Build history of the part. All positions in model axes, mm. Face numbers are marked on the shaded views. A direction names the side the tool comes from. Coordinates: 2 decimals unless noted, no trailing zeros. Loops run counter-clockwise (first coordinate to the right, second up) from the corner with the lowest first, then second, coordinate; pieces in that order, holes last.
(1) Tool access for the marked faces 1, 2 and 3: list every direction of +Z, -Z, +X, -X, +Y, -Y with a clear straight run to the whole face (end or side of a thin tool).
(2) Wall check: L1, parallel to X at y = -52, z = -4; L2, parallel to Z at x = 43, y = -9.5; L3, parallel to Y at x = -4, z = -12.75. Give the ranges that are in metal, low to high.
(3) Flat gauge pins, fed straight in: P1, Ø6, axis at y = -30.5, z = -7.5, coming from the -X side; P2, Ø6.5, axis at y = 7.5, z = 3.5, coming from the -X side; P3, Ø4, axis at x = 3, z = -16.5, coming from the -Y side. Where does each tip first touch, or does it go through?
(4) Slice it at B-B (y = -33). Give the cut face in (x, z) (1 decimal), and give its area (3 significant figures).
(5) Slice it at A-A (x = 1). Give the cut face in (y, z).
(6) Slice it at C-C (z = 3.25). Give the cut face in (x, y) (3 decimals), and give its area (3 significant figures).
(7) Slice it at D-D (z = -16.25). Give the cut face in (x, y), and give its area (3 significant figures).
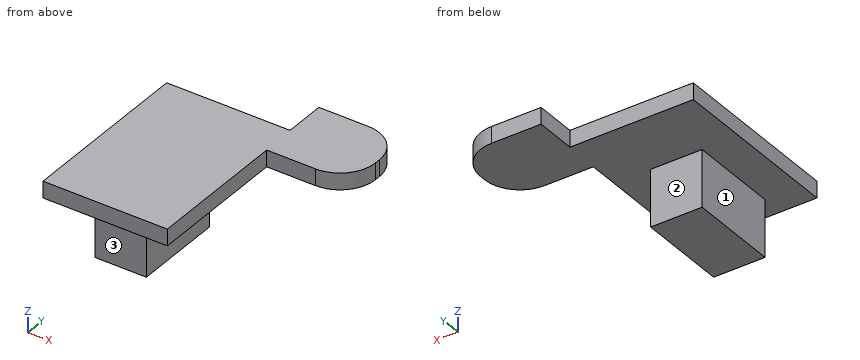
from build123d import *

# Parameters (mm, degrees)
F2_DEPTH = 5.9182
F0_W     = 44.45
F0_H     = 63.5
F3_DEPTH = 5.9182
F4_W     = 18.415
F4_H     = 32.385
F5_DEPTH = 20.32


with BuildPart() as f2:
    # F1 (on Top) → F2 (new body)
    with BuildSketch(Plane.XY):
        with BuildLine():
            Line((39.6100495338, 16.1036532372), (21.8759961426, 16.1036532372))
            Line((21.8759961426, 16.1036532372), (21.8759961426, -11.2066548318))
            Line((21.8759961426, -11.2066548318), (39.6100495338, -11.2066548318))
            ThreePointArc((39.6100495338, -11.2066548318), (48.5903056549, -7.4869109528), (52.3100495338, 1.4933451682))
            Line((52.3100495338, 1.4933451682), (52.3100495338, 3.4036532372))
            ThreePointArc((52.3100495338, 3.4036532372), (48.5903056549, 12.3839093583), (39.6100495338, 16.1036532372))
        make_face()
    extrude(amount=F2_DEPTH)

    # F0 (on Top) + F2_face (on face) → F3 (join)
    with BuildSketch(Plane.XY):
        with Locations((0, -30.48)):
            Rectangle(F0_W, F0_H)
    with BuildSketch(Plane(origin=(35.9682073334, 2.4484992027, 0), x_dir=(1, 0, 0), z_dir=(0, 0, -1))):
        with BuildLine():
            Line((-14.0922111908, -13.6551540345), (3.6418422005, -13.6551540345))
            ThreePointArc((3.6418422005, -13.6551540345), (12.6220983215, -9.9354101556), (16.3418422005, -0.9551540345))
            Line((16.3418422005, -0.9551540345), (16.3418422005, 0.9551540345))
            ThreePointArc((16.3418422005, 0.9551540345), (12.6220983215, 9.9354101556), (3.6418422005, 13.6551540345))
            Line((3.6418422005, 13.6551540345), (-14.0922111908, 13.6551540345))
            Line((-14.0922111908, 13.6551540345), (-14.0922111908, -13.6551540345))
        make_face()
    extrude(amount=F3_DEPTH, dir=(0, 0, 1))

    # F4 (on Top) → F5 (join)
    with BuildSketch(Plane.XY):
        with Locations((0, -38.1122922906)):
            Rectangle(F4_W, F4_H)
    extrude(amount=-F5_DEPTH)


solid = f2.part
Response values:
1. face 1: -Z, -X, +Y, -Y
1. face 2: -Z, +X, -X, +Y
1. face 3: -Z, +X, -X, -Y
2. L1: x = -9.21 to 9.21
2. L2: z = 0 to 5.92
2. L3: y = -54.3 to -21.92
3. P1: stops at x = -9.21
3. P2: stops at x = 21.88
3. P3: stops at y = -54.3
4. outline: (-22.2, 0) - (-9.2, 0) - (-9.2, -20.3) - (9.2, -20.3) - (9.2, 0) - (22.2, 0) - (22.2, 5.9) - (-22.2, 5.9) - close
4. area: 637 mm2
5. outline: (-62.23, 0) - (-54.3, 0) - (-54.3, -20.32) - (-21.92, -20.32) - (-21.92, 0) - (1.27, 0) - (1.27, 5.92) - (-62.23, 5.92) - close
6. outline: (-22.225, -62.23) - (22.225, -62.23) - (22.225, -11.207) - (39.61, -11.207) arc R12.7 ccw to (52.31, 1.493) - (52.31, 3.404) arc R12.7 ccw to (39.61, 16.104) - (21.876, 16.104) - (21.876, 1.27) - (-22.225, 1.27) - close
6. area: 3,580 mm2
7. outline: (-9.21, -54.3) - (9.21, -54.3) - (9.21, -21.92) - (-9.21, -21.92) - close
7. area: 596 mm2
